from build123d import *

# Parameters (mm, degrees)
BOSS_EXTRUDE1_START            = -3
BOSS_EXTRUDE1_OUTLINE_R        = 2.5
BOSS_EXTRUDE1_DEPTH            = 3
FILLET1_R                      = 10
BOSS_EXTRUDE2_START            = -3
BOSS_EXTRUDE2_DEPTH            = 3
CUT_EXTRUDE1_START             = -3
CUT_EXTRUDE1_DEPTH             = 3
FILLET2_R                      = 10
F_2_3_2_3_DIAMETER_HOLE1_D     = 2.3
F_2_3_2_3_DIAMETER_HOLE1_DEPTH = 10
F_2_3_2_3_DIAMETER_HOLE1_TIP   = 0.690989712
SKETCH6_R                      = 5
CUT_EXTRUDE2_DEPTH             = 103.947966144


with BuildPart() as part:
    # Boss-Extrude1: read off the stored shape, not the designer's step
    # Boss-Extrude1 outline → Boss-Extrude1 (new body)
    with BuildSketch(Plane.XY.offset(3).offset(BOSS_EXTRUDE1_START)):
        with BuildLine():
            ThreePointArc((-24.364065342, 16.876742294), (-25.101814907, 17.696096192), (-26.161653435, 18))
            Line((-26.161653435, 18), (-27.830556346, 18))
            ThreePointArc((-27.830556346, 18), (-29.526652538, 17.059838528), (-29.628144438, 15.123257706))
            Line((-29.628144438, 15.123257706), (-16.550964109, -11.68893536))
            ThreePointArc((-16.550964109, -11.68893536), (-15.603505287, -14.937815984), (-15.793938159, -18.316667689))
            Line((-15.793938159, -18.316667689), (-24.617449619, -56.633968709))
            ThreePointArc((-24.617449619, -56.633968709), (-12.550978841, -74.781492041), (4.900124379, -61.728089553))
            Line((4.900124379, -61.728089553), (7.520756747, -39.132184047))
            Line((7.520756747, -39.132184047), (57.484416951, -6.361887987))
            ThreePointArc((57.484416951, -6.361887987), (61.581724267, 4.861915454), (52, 12))
            Line((52, 12), (41.720733512, 12))
            ThreePointArc((41.720733512, 12), (27.868275115, 8.610324995), (17.146172183, -0.792706909))
            Line((17.146172183, -0.792706909), (11.877704642, -8.316858327))
            ThreePointArc((11.877704642, -8.316858327), (-1.137656888, -14.455301339), (-13.032513671, -6.356381628))
            Line((-13.032513671, -6.356381628), (-24.364065342, 16.876742294))
        make_face()
        with Locations((-10, -60)):
            Circle(BOSS_EXTRUDE1_OUTLINE_R, mode=Mode.SUBTRACT)
    extrude(amount=BOSS_EXTRUDE1_DEPTH)

    # Fillet1
    fillet1_edges = [part.edges().sort_by_distance(p)[0] for p in [
        (7.520756747, -39.132184047, 1.5),
    ]]
    fillet(fillet1_edges, radius=FILLET1_R)

    # Sketch2 → Boss-Extrude2 (add)
    with BuildSketch(Plane.XY.offset(3).offset(BOSS_EXTRUDE2_START)):
        with BuildLine():
            Line((11.431019345, -36.567510792), (71.720733512, -18))
            ThreePointArc((71.720733512, -18), (69.105682696, -5.749915992), (61.716429632, 4.364528537))
            ThreePointArc((61.716429632, 4.364528537), (61.302173782, -1.670090316), (57.484416951, -6.361887987))
            Line((57.484416951, -6.361887987), (11.431019345, -36.567510792))
        make_face()
    extrude(amount=BOSS_EXTRUDE2_DEPTH)

    # Sketch2<4> → Cut-Extrude1 (cut)
    with BuildSketch(Plane.XY.offset(3).offset(CUT_EXTRUDE1_START)):
        with BuildLine():
            ThreePointArc((41.720733512, 12), (52.42269931, 10.026200742), (61.716429632, 4.364528537))
            ThreePointArc((61.716429632, 4.364528537), (58.178782835, 9.862737607), (52, 12))
            Line((52, 12), (41.720733512, 12))
        make_face()
    extrude(amount=CUT_EXTRUDE1_DEPTH, mode=Mode.SUBTRACT)

    # Fillet2
    fillet2_edges = [part.edges().sort_by_distance(p)[0] for p in [
        (71.720733512, -18, 1.5),
    ]]
    fillet(fillet2_edges, radius=FILLET2_R)

    # Ø2.3 (2.3) Diameter Hole1
    with Locations(Plane.XY.offset(3)):
        with Locations((-20.357910666, -61.721536128), (-11.721536128, -49.642089334), (-8.278463872, -70.357910666), (0.357910666, -58.278463872)):
            Hole(F_2_3_2_3_DIAMETER_HOLE1_D / 2, depth=F_2_3_2_3_DIAMETER_HOLE1_DEPTH)
            with Locations((0, 0, -(F_2_3_2_3_DIAMETER_HOLE1_DEPTH + F_2_3_2_3_DIAMETER_HOLE1_TIP / 2))):  # 118° drill point
                Cone(0, F_2_3_2_3_DIAMETER_HOLE1_D / 2, F_2_3_2_3_DIAMETER_HOLE1_TIP, mode=Mode.SUBTRACT)

    # Sketch6 → Cut-Extrude2 (cut, through all)
    with BuildSketch(Plane.XY.offset(3)):
        with Locations((-10, -60)):
            Circle(SKETCH6_R)
    extrude(amount=-CUT_EXTRUDE2_DEPTH, mode=Mode.SUBTRACT)


solid = part.part
The listing builds one solid part. Answer for the finished solid, in the listing's coordinates (mm). A direction names the side the tool comes from. Give positions to 0.01 mm unless a question says otherwise; leave off trailing zeros. Write each loop counter-clockwise with the first axis right and the second up, starting at its lowest first coordinate (ties: lowest second). Pieces come first, ordered by that corner, then holes. Notation, with made-up numbers: (84, 22.25) -> (111, 22.25) arc R14 cw to (111, 26.25) -> close; hole circle Ø9 at (82, 48). An arc over 180 degrees is marked (long way). One line per question, with ' | ' between items. Start each with the question number.
1. Section C-C (y = -32.5) is taken. Determine the outline of the cut face in (x, z).
2. Given pin 1 Ø1.4 at (x, y) = (-8.28, -70.36) entering from +Z (3 decimals); pin 2 Ø1 at (y, z) = (-65, 1.5) entering from +X; pin 3 Ø1 at (x, z) = (2.5, 1) entering from -Y, each flat-ended and moving along its own axis, determine where each tip first touches the part or whether it passes through.
3. Find the intervals of material crossed by probe 1 along X at (y, z) = (-50, 2.2); probe 2 along X at (y, z) = (-2.5, 1.1); probe 3 along Y at (x, z) = (-10, 1.65), in increasing order.
4. For a pull along Y with two mould halves and no side action, classify faces 1 (the cylindrical face through (8.438, -39.626, 1.521)), 2 (the cylindrical face through (69.38, -15.52, 1.52)), 3 (the cylindrical face through (0.61, -59.4, 1.48)) as pulls with the +Y half, pulls with the -Y half, needs draft (parallel to the pull), parting line crosses it, or undercut.
5. Section B-B (x = 48) is taken. Determine the outline of the cut face in (y, z).
6. For faces 4 (the flat face through (-20.144, -37.207, 1.479)), 5 (the flat face through (14.55, -4.5, 1.48)), 6 (the flat face through (20, -28, 0)), determine the directions among +Z, -Z, +X, -X, +Y, -Y from which every point of the face is accessible in a straight line to the end or side of a thin tool.
7. Section A-A (z = 2.4) is taken. Determine the outline of the cut face in (x, y).
Response values:
1) outline: (-19.06, 0) -> (24.64, 0) -> (24.64, 3) -> (-19.06, 3) -> close
2) pin 1: through | pin 2: x = 4.31 | pin 3: y = -69
3) probe 1: -23.09 to -12.81, -10.63 to 6.26 | probe 2: -21.03 to -14.91, 15.95 to 67.41 | probe 3: -75 to -65, -55 to -10.5
4) face 1: pulls with the -Y half | face 2: parting line crosses it | face 3: undercut
5) outline: (-25.31, 0) -> (11.34, 0) -> (11.34, 3) -> (-25.31, 3) -> close
6) face 4: +Z, -Z, -X | face 5: +Z, -Z, +Y | face 6: -Z, +X, -X, +Y, -Y
7) outline: (-29.63, 15.12) -> (-16.55, -11.69) arc R10 cw to (-15.79, -18.32) -> (-24.62, -56.63) arc R15 ccw (long way) to (4.9, -61.73) -> (6.98, -43.78) arc R10 cw to (11.43, -36.57) -> (63.4, -20.56) arc R10 ccw to (69.83, -7.51) arc R30 ccw to (17.15, -0.79) -> (11.88, -8.32) arc R14.5 cw to (-13.03, -6.36) -> (-24.36, 16.88) arc R2 ccw to (-26.16, 18) -> (-27.83, 18) arc R2 ccw to start; hole circle Ø2.3 at (-20.36, -61.72); hole circle Ø10 at (-10, -60); hole circle Ø2.3 at (-11.72, -49.64); hole circle Ø2.3 at (-8.28, -70.36); hole circle Ø2.3 at (0.36, -58.28)
